from build123d import *

# Parameters (mm, degrees)
F0_W      = 760
F0_H      = 360
F1_DEPTH  = 1.5
F2_W      = 20
F2_H      = 20
F3_DEPTH  = 3.001
F4_R      = 1.55
F5_DEPTH  = 3.001
F6_W      = 50
F6_H      = 20
F7_DEPTH  = 3.001
F8_R      = 1.55
F9_DEPTH  = 3.001
F10_W     = 40
F10_H     = 4
F11_DEPTH = 3.001
F12_W     = 760
F12_H     = 160
F13_DEPTH = 3.001


with BuildPart() as f1:
    # F0 (on Top) → F1 (new body, symmetric)
    with BuildSketch(Plane.XY):
        Rectangle(F0_W, F0_H)
    extrude(amount=F1_DEPTH, both=True)

    # F2 (on face) → F3 (cut, through all)
    with BuildSketch(Plane.XY.offset(1.5)):
        with Locations((-370, -170)):
            Rectangle(F2_W, F2_H)
        with Locations((-370, 170)):
            Rectangle(F2_W, F2_H)
        with Locations((370, -170)):
            Rectangle(F2_W, F2_H)
        with Locations((370, 170)):
            Rectangle(F2_W, F2_H)
    extrude(amount=-F3_DEPTH, mode=Mode.SUBTRACT)

    # F4 (on face) → F5 (cut, through all)
    with BuildSketch(Plane.XY.offset(1.5)):
        with Locations((-370.5, 145)):
            Circle(F4_R)
        with Locations((-370.5, 0)):
            Circle(F4_R)
        with Locations((-370.5, -145)):
            Circle(F4_R)
        with Locations((370.5, -145)):
            Circle(F4_R)
        with Locations((370.5, 0)):
            Circle(F4_R)
        with Locations((370.5, 145)):
            Circle(F4_R)
        with Locations((0, 170.5)):
            Circle(F4_R)
        with Locations((172.5, 170.5)):
            Circle(F4_R)
        with Locations((345, 170.5)):
            Circle(F4_R)
        with Locations((-172.5, 170.5)):
            Circle(F4_R)
        with Locations((-345, 170.5)):
            Circle(F4_R)
        with Locations((-345, -170.5)):
            Circle(F4_R)
        with Locations((-172.5, -170.5)):
            Circle(F4_R)
        with Locations((0, -170.5)):
            Circle(F4_R)
        with Locations((172.5, -170.5)):
            Circle(F4_R)
        with Locations((345, -170.5)):
            Circle(F4_R)
    extrude(amount=-F5_DEPTH, mode=Mode.SUBTRACT)

    # F6 (on face) → F7 (cut, through all)
    with BuildSketch(Plane.XY.offset(1.5)):
        with Locations((-234.763, 110)):
            Rectangle(F6_W, F6_H)
        with Locations((-143.659, 110)):
            Rectangle(F6_W, F6_H)
        with Locations((-52.555, 110)):
            Rectangle(F6_W, F6_H)
        with Locations((125, 110)):
            Rectangle(F6_W, F6_H)
        with Locations((225, 110)):
            Rectangle(F6_W, F6_H)
        with Locations((325, 110)):
            Rectangle(F6_W, F6_H)
        with Locations((20, 110)):
            Rectangle(F6_W, F6_H)
        with Locations((-325.867, 110)):
            Rectangle(F6_W, F6_H)
    extrude(amount=-F7_DEPTH, mode=Mode.SUBTRACT)

    # F8 (on face) → F9 (cut, through all)
    with BuildSketch(Plane.XY.offset(1.5)):
        with Locations((-341.6325, -16)):
            Circle(F8_R)
        with Locations((-306.6325, -16)):
            Circle(F8_R)
        with Locations((-341.6325, -112)):
            Circle(F8_R)
        with Locations((-306.6325, -112)):
            Circle(F8_R)
        with Locations((-252.263, -112)):
            Circle(F8_R)
        with Locations((-217.263, -112)):
            Circle(F8_R)
        with Locations((-252.263, -16)):
            Circle(F8_R)
        with Locations((-217.263, -16)):
            Circle(F8_R)
        with Locations((-162.893, -16)):
            Circle(F8_R)
        with Locations((-127.893, -16)):
            Circle(F8_R)
        with Locations((-162.893, -112)):
            Circle(F8_R)
        with Locations((-127.893, -112)):
            Circle(F8_R)
        with Locations((-73.523, -112)):
            Circle(F8_R)
        with Locations((-38.523, -112)):
            Circle(F8_R)
        with Locations((-73.523, -16)):
            Circle(F8_R)
        with Locations((-38.523, -16)):
            Circle(F8_R)
        with Locations((15.847, -16)):
            Circle(F8_R)
        with Locations((50.847, -16)):
            Circle(F8_R)
        with Locations((15.847, -112)):
            Circle(F8_R)
        with Locations((50.847, -112)):
            Circle(F8_R)
        with Locations((105.217, -112)):
            Circle(F8_R)
        with Locations((140.217, -112)):
            Circle(F8_R)
        with Locations((105.217, -16)):
            Circle(F8_R)
        with Locations((140.217, -16)):
            Circle(F8_R)
        with Locations((194.587, -16)):
            Circle(F8_R)
        with Locations((229.587, -16)):
            Circle(F8_R)
        with Locations((194.587, -112)):
            Circle(F8_R)
        with Locations((229.587, -112)):
            Circle(F8_R)
        with Locations((283.957, -112)):
            Circle(F8_R)
        with Locations((318.957, -112)):
            Circle(F8_R)
        with Locations((283.957, -16)):
            Circle(F8_R)
        with Locations((318.957, -16)):
            Circle(F8_R)
    extrude(amount=-F9_DEPTH, mode=Mode.SUBTRACT)

    # F10 (on face) → F11 (cut, through all)
    with BuildSketch(Plane.XY.offset(1.5)):
        with Locations((-312.825, -160)):
            Rectangle(F10_W, F10_H)
        with Locations((-223.455, -160)):
            Rectangle(F10_W, F10_H)
        with Locations((-134.085, -160)):
            Rectangle(F10_W, F10_H)
        with Locations((-44.715, -160)):
            Rectangle(F10_W, F10_H)
        with Locations((44.655, -160)):
            Rectangle(F10_W, F10_H)
        with Locations((134.025, -160)):
            Rectangle(F10_W, F10_H)
        with Locations((223.395, -160)):
            Rectangle(F10_W, F10_H)
        with Locations((312.765, -160)):
            Rectangle(F10_W, F10_H)
    extrude(amount=-F11_DEPTH, mode=Mode.SUBTRACT)

    # F12 (on face) → F13 (cut, through all)
    with BuildSketch(Plane.XY.offset(1.5)):
        with Locations((0, 100)):
            Rectangle(F12_W, F12_H)
    extrude(amount=-F13_DEPTH, mode=Mode.SUBTRACT)


solid = f1.part
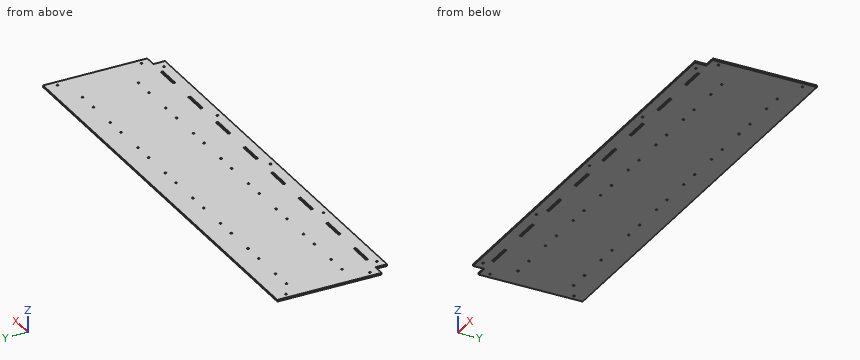
CAD build for the part. Positions are in the model's coordinates, mm. Round coordinates to 2 decimals unless told otherwise and drop trailing zeros. Answer as a JSON object with one key per item and string values.
(1) Probe probe 1 along Y at (x, z) = (370.5, 0.9); probe 2 along Y at (x, z) = (300, 1); probe 3 along Y at (x, z) = (345, -0.6). List the from-to ranges inside material, lowest first. Write a range as [from, to].
Reported:
{"probe 1": "y = [-160, -146.55], [-143.45, -1.55], [1.55, 20]", "probe 2": "y = [-180, -162], [-158, 20]", "probe 3": "y = [-180, -172.05], [-168.95, 20]"}
(2) Band-saw the part on A-A, the plane z = 0.4. Count the separate pieces of the cut face and the enclosed holes in it, then the cut area to 3 significant figures.
Reported:
{"separate pieces": "1", "enclosed holes": "49", "area": "150,000 mm^2"}
(3) Pin check, flat tip, straight feed: P1, Ø2.5, axis at x = 15.847, y = -112, coming from the -Z side. Stop position of the tip, or through.
Reported:
{"P1": "passes through"}
